Autodesk Inventor part; units mm, degrees
ref_plane "YZ Plane" through (0, 0, 0) normal (1, 0, 0) x (0, 1, 0)
ref_plane "XZ Plane" through (0, 0, 0) normal (0, 1, 0) x (-1, 0, 0)
ref_plane "XY Plane" through (0, 0, 0) normal (0, 0, 1) x (1, 0, 0)
sketch "Эскиз1" plane through (0, 0, 0) normal (0, 0, 1) x (1, 0, 0)
  circle A0 centre (0, 0) radius 1.35
  line L0 (0, 3.1292) -> (2.71, 1.5646)
  line L1 (2.71, 1.5646) -> (2.71, -1.5646)
  line L2 (2.71, -1.5646) -> (0, -3.1292)
  line L3 (0, -3.1292) -> (-2.71, -1.5646)
  line L4 (-2.71, -1.5646) -> (-2.71, 1.5646)
  line L5 (-2.71, 1.5646) -> (0, 3.1292)
  dimension "d0" = 2.7
  dimension "d1" = 5.42
extrude "Выдавливание1" add sketch "Эскиз1" along normal mid plane 2.4
chamfer "Фаска1" distance 0.4 angle 45 2 edges at (-1.35, 0, 1.2) (-1.35, 0, -1.2)
sketch "Эскиз2" plane through (0, 0, 0) normal (1, 0, 0) x (0, 1, 0)
  line L0 (0, -4.7585) -> (0, 2.7781)
  line L1 (3.1292, -1.2) -> (3.1292, 1.2)
  line L2 (1.5646, 1.2) -> (3.1292, 1.2)
  line L3 (1.5646, -1.2) -> (1.5646, 1.2)
  line L4 (3.1292, -1.2) -> (1.5646, -1.2)
  line L5 (3.1292, 0.8083) -> (2.4508, 1.2)
  point P0 (0, 0)
  dimension "d7" = 30
revolve "Вращение1" cut sketch "Эскиз2" angle 360 about axis through (0, 0, -4.7585) along (0, 0, 1) contours L5 L2 L1
mirror "Зеркальное отражение1" about plane through (0, 0, 0) normal (0, 0, 1) of "Вращение1"
properties part number "Гайка М3"
The listing builds one solid part. Answer for the finished solid, in the listing's coordinates (mm). Round coordinates to 2 decimals unless told otherwise and drop trailing zeros. Order: outer loops, then holes, each group sorted by start corner. A loop starts at its lowest first (then second) coordinate and runs counter-clockwise, first axis right, second up. Notation, with made-up numbers: (5.25, 50.25) - (43.25, 50.25) arc R33 ccw to (43.25, 87.25) - close; hole circle Ø7 at (13, -4.75). An arc over 180 degrees is marked (long way). Write item = value, one per line. Start each with the question number.
1) Given pin 1 (2 mm diameter, centred on x = 0.5, y = -1.5, fed in from -Z), flat-ended and moving along its own axis, determine where the tip first touches the part or whether it passes through.
2) Section A-A, the plane y = 0 is taken. Write down the section's boundary in (x, z), plus the area to 3 significant figures.
3) Section B-B, the plane z = 0.9 is taken. Write down the section's boundary in (x, y).
4) For a pull along Y with two mould halves and no side action, classify faces 1 (the flat face through (-2, 1, 1.2)), 2 (the flat face through (-1.336, -2.358, -0.015)), 3 (the cylindrical face through (-0.29, 1.32, -0.01)), 4 (the flat face through (-1.37, 2.34, -0.01)) as released by +Y, released by -Y, zero draft, split by the parting line, or undercut.
5) Straight lines are drawn through the part: L1, parallel to Z at x = -0.55, y = -1.5; L2, parallel to Y at x = -1.25, z = -1; L3, parallel to Y at x = -0.5, z = 0.3. For each, find the intervals that lie inside material, in ascending order.
6) Section C-C, the plane z = 0.4 is taken. Write down the section's boundary in (x, y), plus the area to 3 significant figures.
Results list:
q1.pin_1 = -1.2
q2.outline = (-2.71, -1.05) - (-2.45, -1.2) - (-1.75, -1.2) - (-1.35, -0.8) - (-1.35, 0.8) - (-1.75, 1.2) - (-2.45, 1.2) - (-2.71, 1.05) - close; (1.35, -0.8) - (1.75, -1.2) - (2.45, -1.2) - (2.71, -1.05) - (2.71, 1.05) - (2.45, 1.2) - (1.75, 1.2) - (1.35, 0.8) - close
q2.area = 6.13 mm^2
q3.outline = (-2.71, -1.22) arc R2.97 ccw to (-2.41, -1.74) - (-0.3, -2.96) arc R2.97 ccw to (0.3, -2.96) - (2.41, -1.74) arc R2.97 ccw to (2.71, -1.22) - (2.71, 1.22) arc R2.97 ccw to (2.41, 1.74) - (0.3, 2.96) arc R2.97 ccw to (-0.3, 2.96) - (-2.41, 1.74) arc R2.97 ccw to (-2.71, 1.22) - close; hole circle Ø2.9 at (0, 0)
q4.face_1 = zero draft
q4.face_2 = released by -Y
q4.face_3 = undercut
q4.face_4 = released by +Y
q5.L1 = -1.05 to 1.05
q5.L2 = -2.41 to -0.92, 0.92 to 2.41
q5.L3 = -2.84 to -1.25, 1.25 to 2.84
q6.outline = (-2.71, -1.56) - (0, -3.13) - (2.71, -1.56) - (2.71, 1.56) - (0, 3.13) - (-2.71, 1.56) - close; hole circle Ø2.7 at (0, 0)
q6.area = 19.7 mm^2
